Verification items for the finished model (mm, model axes). Face numbers are marked on the shaded views. A direction names the side the tool comes from. Round coordinates to 2 decimals unless told otherwise and drop trailing zeros. Order: outer loops, then holes, each group sorted by start corner. A loop starts at its lowest first (then second) coordinate and runs counter-clockwise, first axis right, second up. Notation, with made-up numbers: (-15.5, -38.5) -> (-6.5, -38.5) arc R23 cw to (-6.5, -6.5) -> close; hole circle Ø7 at (70, 48). An arc over 180 degrees is marked (long way). Put each result on its own line as item: value.
```python
from build123d import *

# Parameters (mm, degrees)
F0_R     = 11
F1_DEPTH = 3.5
F2_R     = 5
F3_DEPTH = 1
F4_R     = 4
F5_DEPTH = 3.5
F6_R     = 1.3518679975
F7_DEPTH = 32.3
F11_R    = 0.9092071391


# Not quite as in the source:
# - a fillet or chamfer that OpenCascade refuses, or shapes differently, is made with other operations: its cross-section is extruded or revolved along the edge and cut away or added
# - a feature names something its author has since deleted; it is built from what else it names


with BuildPart() as f1:
    # F0 (on Top) → F1 (new body)
    with BuildSketch(Plane.XY):
        with Locations((59.4149753451, 64.0600547194)):
            Circle(F0_R)
    extrude(amount=F1_DEPTH)

    # F2 (on face) → F3 (join)
    with BuildSketch(Plane.XY.offset(3.5)):
        with Locations((59.4149753451, 64.0600547194)):
            Circle(F2_R)
    extrude(amount=F3_DEPTH)

    # F4 (on face) → F5 (join)
    with BuildSketch(Plane.XY.offset(4.5)):
        with Locations((59.4149753451, 64.0600547194)):
            Circle(F4_R)
    extrude(amount=F5_DEPTH)

    # F6 (on face) → F7 (join)
    with BuildSketch(Plane(origin=(0, 0, 0), x_dir=(1, 0, 0), z_dir=(0, 0, -1))):
        with Locations((59.4149753451, -64.0600547194)):
            Circle(F6_R)
    extrude(amount=F7_DEPTH)

    # F8 (on face) → F9 (revolve, cut)
    with BuildSketch(Plane(origin=(0, 0, -32.3), x_dir=(1, 0, 0), z_dir=(0, 0, -1))):
        with BuildLine():
            Line((60.7668433426, -64.0600547194), (93.4149753451, -64.0600547194))
            ThreePointArc((93.4149753451, -64.0600547194), (59.4149753451, -30.0600547194), (25.4149753451, -64.0600547194))
            Line((25.4149753451, -64.0600547194), (58.0631073476, -64.0600547194))
            ThreePointArc((58.0631073476, -64.0600547194), (59.4149753451, -62.7081867219), (60.7668433426, -64.0600547194))
        make_face()
        with BuildLine():
            Line((59.4149753451, -64.0600547194), (60.7668433426, -64.0600547194))
            ThreePointArc((60.7668433426, -64.0600547194), (59.4149753451, -62.7081867219), (58.0631073476, -64.0600547194))
            Line((58.0631073476, -64.0600547194), (59.4149753451, -64.0600547194))
        make_face()
    revolve(axis=Axis((76.4149753451, 64.0600547194, -32.3), (1, 0, 0)), mode=Mode.SUBTRACT)

    # F10: fillet of radius 5 on 1 edges, made by hand

    # F10_s1 → F10_t2 (revolve, cut)
    with BuildSketch(Plane.YZ.offset(59.4149753451)):
        with BuildLine():
            ThreePointArc((52.67102491, 0), (53.4091792265, 0.0547873448), (54.1311569369, 0.2179487179))
            ThreePointArc((54.1311569369, 0.2179487179), (53.7867795374, 0.1107978463), (53.4435581222, 0))
            Line((53.4435581222, 0), (52.67102491, 0))
        make_face()
    revolve(axis=Axis((59.4149753451, 64.0600547194, 0), (0, 0, 1)), mode=Mode.SUBTRACT)

    # F11
    f11_edges = [f1.edges().sort_by_distance(p)[0] for p in [
        (51.636801, 71.838229, 0.015157),
        (67.19315, 56.28188, 0.015157),
    ]]
    fillet(f11_edges, radius=F11_R)


solid = f1.part
```
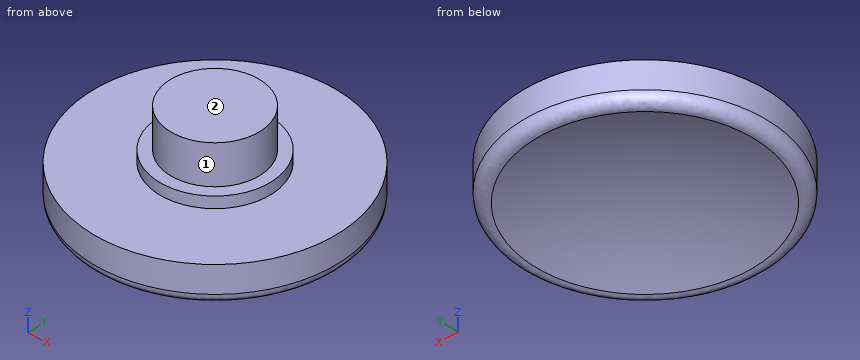
Item 1: Depth check by flat-ended pin: pin 1 Ø1 at (x, z) = (53, 1) entering from -Y; pin 2 Ø3 at (y, z) = (67.5, 4) entering from +X; pin 3 Ø2 at (y, z) = (56.5, 5.5) entering from +X; pin 4 Ø2 at (y, z) = (61, 7) entering from -X. Enter the tip coordinate at first touch or a pass-through.
Geometry check:
pin 1: y = 54.79
pin 2: x = 70.23
pin 3: through
pin 4: x = 55.99
Item 2: Material ranges on line 1 along Z through (x, y) = (69.5, 65.5); line 2 along X through (y, z) = (65.25, 6.25); line 3 along X through (y, z) = (61.75, 7.75), recorded low to high.
Geometry check:
line 1: 0.21 to 3.5
line 2: 55.6 to 63.23
line 3: 56.15 to 62.68
Item 3: Sectioned sample at B-B, the plane z = 3. Record the boundary of the cut face in (x, y).
Geometry check:
outline: circle Ø22 at (59.41, 64.06)
Item 4: Sectioned sample at A-A, the plane z = 6. Record the boundary of the cut face in (x, y), then the cut area to 3 significant figures.
Geometry check:
outline: circle Ø8 at (59.41, 64.06)
area: 50.3 mm2
Item 5: Tool access check on the marked faces 1 and 2. Record the directions out of +Z, -Z, +X, -X, +Y, -Y that give a thin tool (end or side, any length) a straight path to the whole face; none if there is none.
Geometry check:
face 1: +Z
face 2: +Z, +X, -X, +Y, -Y
